```python
from build123d import *

# Parameters (mm, degrees)
F1_DEPTH = 6.35


# Not quite as in the source:
# - a length typed as a fraction of an inch, garbled in the dataset ("3 / 203.2 mm" for 3/8 in), is restored


with BuildPart() as f1:
    # F0 (on Top) → F1 (new body)
    with BuildSketch(Plane.XY):
        with BuildLine():
            ThreePointArc((0, 7.5), (-7.5, 0), (0, -7.5))
            ThreePointArc((0, -7.5), (11.25, -10.5144284149), (19.4855715851, -18.75))
            ThreePointArc((19.4855715851, -18.75), (29.7307621135, -21.4951905284), (32.4759526419, -11.25))
            ThreePointArc((32.4759526419, -11.25), (18.75, 2.4759526419), (0, 7.5))
        make_face()
        with BuildLine():
            ThreePointArc((2.4978289184, -0.1041666667), (-2.4994571707, 0.0520946447), (2.5, 0))
            ThreePointArc((2.5, 0), (2.4994571707, -0.0520946447), (2.4978289184, -0.1041666667))
        make_face(mode=Mode.SUBTRACT)
    extrude(amount=F1_DEPTH)


solid = f1.part
```
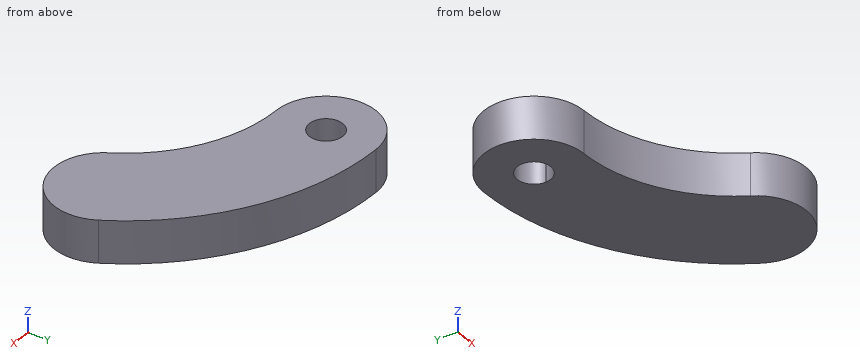
Part model, mm, in its own coordinate system. Give positions to 0.01 mm unless a question says otherwise; leave off trailing zeros. Order: outer loops, then holes, each group sorted by start corner. A loop starts at its lowest first (then second) coordinate and runs counter-clockwise, first axis right, second up. Notation, with made-up numbers: (50, 81.25) - (99, 81.25) arc R14 ccw to (99, 101.25) - close; hole circle Ø7 at (-8.75, -25.75). An arc over 180 degrees is marked (long way). Use one line per item in the form item = value.
Item 1: Slice it at A-A on z = 2. Give the cut face in (x, y).
Solution:
outline = (0, -7.5) arc R22.5 cw to (19.49, -18.75) arc R7.5 ccw to (32.48, -11.25) arc R37.5 ccw to (0, 7.5) arc R7.5 ccw to start; hole circle Ø5 at (0, 0)
Item 2: Slice it at D-D on x = 26. Give the cut face in (y, z), and give its area (3 significant figures).
Solution:
outline = (-22.5, 0) - (-2.98, 0) - (-2.98, 6.35) - (-22.5, 6.35) - close
area = 124 mm2
Item 3: Slice it at B-B on x = -2. Give the cut face in (y, z).
Solution:
outline = (-7.23, 0) - (-1.5, 0) - (-1.5, 6.35) - (-7.23, 6.35) - close; (1.5, 0) - (7.23, 0) - (7.23, 6.35) - (1.5, 6.35) - close
Item 4: Probe probe 1 along Y at (x, z) = (0, 2); probe 2 along X at (y, z) = (0, 4); probe 3 along Y at (x, z) = (1, 5.25). List the from-to ranges inside material, lowest first. Write a range as from..to.
Solution:
probe_1 = -7.5..-2.5, 2.5..7.5
probe_2 = -7.5..-2.5, 2.5..22.5
probe_3 = -7.52..-2.29, 2.29..7.49
Item 5: Slice it at C-C on y = -17. Give the cut face in (x, z).
Solution:
outline = (18.36, 0) - (33.21, 0) - (33.21, 6.35) - (18.36, 6.35) - close
Item 6: Pin check, flat tips, straight feed: pin 1 Ø1 at (y, z) = (-2.5, 4) entering from -X; pin 2 Ø3 at (x, z) = (14.5, 4.5) entering from +Y; pin 3 Ø6 at (x, y) = (1, -2) entering from -Z; pin 4 Ø1.5 at (y, z) = (-4.5, 5) entering from -X. Stop position of each tip, or through.
Solution:
pin_1 = -7.23
pin_2 = 5.17
pin_3 = 0
pin_4 = -6.5
